```python
from build123d import *

# Parameters (mm, degrees)
F0_W     = 67.31
F0_H     = 139.7
F1_DEPTH = 7.62
F2_R     = 5.08
F3_T     = -2.54
F4_R     = 5.08
F6_R     = 5.08
F7_D     = 3.556
F8_D     = 3.556


with BuildPart() as f1:
    # F0 (on Top) → F1 (new body)
    with BuildSketch(Plane.XY):
        Rectangle(F0_W, F0_H)
    extrude(amount=F1_DEPTH)

    # F2
    f2_edges = [f1.edges().sort_by_distance(p)[0] for p in [
        (33.655, 69.85, 3.81),
        (-33.655, 69.85, 3.81),
    ]]
    fillet(f2_edges, radius=F2_R)

    # F3
    f3_openings = [f1.faces().sort_by_distance(p)[0] for p in [
        (0, -0.081036, 7.62),
    ]]
    offset(amount=F3_T, openings=f3_openings)

    # F4
    f4_edges = [f1.edges().sort_by_distance(p)[0] for p in [
        (-33.655, -69.85, 3.81),
    ]]
    fillet(f4_edges, radius=F4_R)

    # F6
    f6_edges = [f1.edges().sort_by_distance(p)[0] for p in [
        (33.655, -69.85, 3.81),
    ]]
    fillet(f6_edges, radius=F6_R)

    # F7 (through all)
    with Locations(Plane(origin=(0, 0, 0), x_dir=(1, 0, 0), z_dir=(0, 0, -1))):
        with Locations((18.2498693466, -64.5460113883)):
            Hole(F7_D / 2)

    # F8 (through all)
    with Locations(Plane(origin=(0, 0, 0), x_dir=(1, 0, 0), z_dir=(0, 0, -1))):
        with Locations((22.9663196951, -64.4813999534)):
            Hole(F8_D / 2)


solid = f1.part
```
CAD build for the part. Positions are in the model's coordinates, mm. A direction names the side the tool comes from. Round coordinates to 2 decimals unless told otherwise and drop trailing zeros. Order: outer loops, then holes, each group sorted by start corner. A loop starts at its lowest first (then second) coordinate and runs counter-clockwise, first axis right, second up. Notation, with made-up numbers: (53.25, 24) -> (93.25, 24) arc R25 cw to (93.25, 43) -> close; hole circle Ø3 at (8, 26.5). An arc over 180 degrees is marked (long way). Write item = value, one per line.
(1) Flat gauge pins, fed straight in: P1, Ø5.5, axis at x = 18.25, y = 64.55, coming from the -Z side; P2, Ø6, axis at x = 13, y = -44.5, coming from the +Z side; P3, Ø2, axis at x = 22.97, y = 64.48, coming from the +Z side. Where does each tip first touch, or does it go through?
Answers follow:
P1 = 0
P2 = 2.54
P3 = through
(2) Drill centre lines: L1, parallel to X at y = -5, z = 3.75 (3 decimals); L2, parallel to Y at x = -18, z = 4.75; L3, parallel to Z at x = 10.5, y = 42. Where is each one in solid material? Low to high.
Answers follow:
L1 = -33.655 to -31.115, 31.115 to 33.655
L2 = -69.85 to -67.31, 67.31 to 69.85
L3 = 0 to 2.54
(3) 3-axis set-ups, long thin cutter, end or side, ignore diameter. For faces 1 (the flat face through (-33.655, -1, 4)), 2 (the cylindrical face through (30.391, 66.546, 5.116)): which of +Z, -Z, +X, -X, +Y, -Y reach the whole face in a straight line?
Answers follow:
face_1 = +Z, -Z, -X, +Y, -Y
face_2 = +Z
(4) Cut at A-A (z = 5.25). Write the cut outline in (x, y) (3 decimals).
Answers follow:
outline = (-33.655, -64.77) arc R5.08 ccw to (-28.575, -69.85) -> (28.575, -69.85) arc R5.08 ccw to (33.655, -64.77) -> (33.655, 64.77) arc R5.08 ccw to (28.575, 69.85) -> (-28.575, 69.85) arc R5.08 ccw to (-33.655, 64.77) -> close; hole (-31.115, -67.31) -> (31.115, -67.31) -> (31.115, 64.77) arc R2.54 ccw to (28.575, 67.31) -> (-28.575, 67.31) arc R2.54 ccw to (-31.115, 64.77) -> close
(5) Pull direction Y, two halves, no side cores. Call faces 3 (the flat face through (31.115, -2, 5)), 4 (the cylindrical face through (-32.21, -68.32, 3.86)), 5 (the flat face through (32, 21, 7.62)), 6 (the cylindrical face through (-32.21, 68.32, 3.86)): +Y half, -Y half, draft (parallel to the pull), parting line (faces both ways), or undercut.
Answers follow:
face_3 = undercut
face_4 = -Y half
face_5 = draft
face_6 = +Y half
(6) Cut at B-B (x = -4). Write the cut outline in (y, z).
Answers follow:
outline = (-69.85, 0) -> (69.85, 0) -> (69.85, 7.62) -> (67.31, 7.62) -> (67.31, 2.54) -> (-67.31, 2.54) -> (-67.31, 7.62) -> (-69.85, 7.62) -> close
(7) Cut at C-C (y = 0). Write the cut outline in (x, z) (3 decimals), plus the area to 3 significant figures.
Answers follow:
outline = (-33.655, 0) -> (33.655, 0) -> (33.655, 7.62) -> (31.115, 7.62) -> (31.115, 2.54) -> (-31.115, 2.54) -> (-31.115, 7.62) -> (-33.655, 7.62) -> close
area = 197 mm²
